Geometry: final body of the model. Coordinates: model frame, mm. Give positions to 0.01 mm unless a question says otherwise; leave off trailing zeros. Order: outer loops, then holes, each group sorted by start corner. A loop starts at its lowest first (then second) coordinate and runs counter-clockwise, first axis right, second up. Notation, with made-up numbers: (65, -18.5) - (76, -18.5) arc R9 ccw to (76, -13.5) - close; hole circle Ø7 at (11, 48). An arc over 180 degrees is marked (long way). Use one line per item in the form item = value.
Autodesk Inventor part; units mm, degrees
ref_plane "YZ Plane" through (0, 0, 0) normal (1, 0, 0) x (0, 1, 0)
ref_plane "XZ Plane" through (0, 0, 0) normal (0, 1, 0) x (-1, 0, 0)
ref_plane "XY Plane" through (0, 0, 0) normal (0, 0, 1) x (1, 0, 0)
sketch "Sketch1" plane through (0, 0, 0) normal (0, 1, 0) x (-1, 0, 0)
  line L0 (0, 0) -> (-58, 0)
  line L1 (-58, 0) -> (-58, -9.5)
  line L2 (-58, -9.5) -> (0, -9.5)
  line L3 (0, -9.5) -> (0, 0)
  dimension "d0" = 58
  dimension "d1" = 9.5
extrude "Extrusion1" add sketch "Sketch1" along normal blind 4.3
fillet "Fillet1" radius 1 12 edges at (0, 0, -4.75) (0, 2.15, 0) (0, 4.3, -4.75) (0, 2.15, -9.5) (29, 0, -9.5) (29, 4.3, -9.5) (58, 2.15, -9.5) (58, 0, -4.75) (58, 4.3, -4.75) (58, 2.15, 0) (29, 0, 0) (29, 4.3, 0)
properties part number "Magnet6010" material "Stainless Steel"
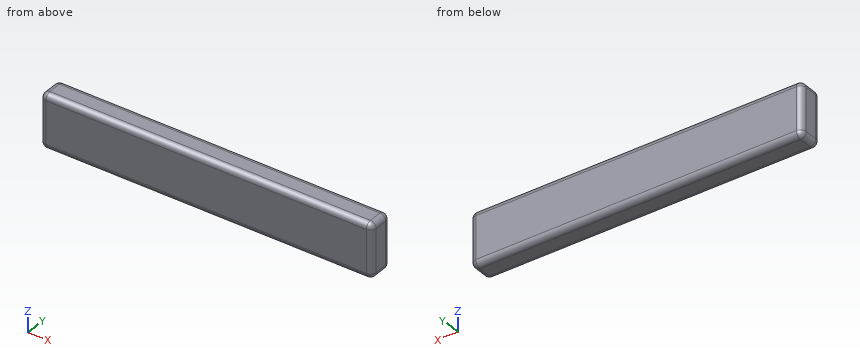
(1) Ray query, line 1 along X through (y, z) = (0.85, -8); line 2 along Z through (x, y) = (47, 3.5); line 3 along Y through (x, z) = (26.5, -0.5). Return the intervals inside material, ascending.
Computed values:
line_1 = 0.01 to 57.99
line_2 = -9.48 to -0.02
line_3 = 0.13 to 4.17
(2) Cut plane B-B on z = -9. Output: boundary loops of the cut face in (x, y), plus the area to 3 significant figures.
Computed values:
outline = (0.13, 1) arc R0.87 ccw to (1, 0.13) - (57, 0.13) arc R0.87 ccw to (57.87, 1) - (57.87, 3.3) arc R0.87 ccw to (57, 4.17) - (1, 4.17) arc R0.87 ccw to (0.13, 3.3) - close
area = 232 mm²
(3) Cut plane A-A on x = 19. Output: boundary loops of the cut face in (y, z), plus the area to 3 significant figures.
Computed values:
outline = (0, -8.5) arc R1 ccw to (1, -9.5) - (3.3, -9.5) arc R1 ccw to (4.3, -8.5) - (4.3, -1) arc R1 ccw to (3.3, 0) - (1, 0) arc R1 ccw to (0, -1) - close
area = 40.0 mm²
